from build123d import *

# Parameters (mm, degrees)
SKETCH1_R           = 3.81
BOSS_EXTRUDE1_DEPTH = 17.2974
SKETCH1_6_R         = 3.175
SKETCH1_6_R_2       = 2.8575
CUT_EXTRUDE1_DEPTH  = 2.54
SKETCH1_7_R         = 1.27
CUT_EXTRUDE2_DEPTH  = 1.27


with BuildPart() as part:
    # Sketch1 → Boss-Extrude1 (new body)
    with BuildSketch(Plane.XY):
        Circle(SKETCH1_R)
    extrude(amount=-BOSS_EXTRUDE1_DEPTH)

    # Sketch1<6> → Cut-Extrude1 (cut)
    with BuildSketch(Plane.XY):
        Circle(SKETCH1_6_R)
        Circle(SKETCH1_6_R_2, mode=Mode.SUBTRACT)
    extrude(amount=-CUT_EXTRUDE1_DEPTH, mode=Mode.SUBTRACT)

    # Sketch1<7> → Cut-Extrude2 (cut)
    with BuildSketch(Plane.XY):
        Circle(SKETCH1_7_R)
    extrude(amount=-CUT_EXTRUDE2_DEPTH, mode=Mode.SUBTRACT)


solid = part.part
The model under review builds one solid part; all positions refer to its coordinate system, in mm. A direction names the side the tool comes from. Give positions to 0.01 mm unless a question says otherwise; leave off trailing zeros. Order: outer loops, then holes, each group sorted by start corner. A loop starts at its lowest first (then second) coordinate and runs counter-clockwise, first axis right, second up. Notation, with made-up numbers: M -10,41.5 L -2,41.5 A20 ccw -2,57.5 Z; hole C 20,81.25 d4. An arc over 180 degrees is marked long. Use one line per item in the form item = value. Start each with the question number.
Item 1: For faces 4 (the cylindrical face through (-0.17, 1.26, -0.63)), 5 (the flat face through (0, 0, -17.297)), list the 3-axis set-ups (+Z, -Z, +X, -X, +Y, -Y) from which the entire face can be reached by the end or side of a thin tool; tool diameter is ignored.
Item 2: To check wall thickness, follow line 1 along Y through (x, z) = (0, -0.6) (1 decimal); line 2 along Y through (x, z) = (0, -1.8) (1 decimal); line 3 along Z through (x, y) = (3, -0.5). State the ranges of each line that lie inside material, in increasing order. Write a range as from..to.
Item 3: We need section D-D on x = 2.5. Give the boundary of the cut face in (y, z), plus the area to 3 significant figures.
Item 4: Insertion check: pin 1 Ø2 at (x, z) = (2, -4) entering from -Y; pin 2 Ø4 at (x, z) = (2.5, -6.5) entering from +Y. Each pin has a flat end and moves straight along its axis. Give the tip position at first contact, or say it passes through.
Item 5: The part is to be moulded in two halves that separate along X. For faces 1 (the cylindrical face through (-0.83, -3.72, -8.53)), 2 (the flat face through (-2, 3, 0)), 3 (the cylindrical face through (-0.69, -3.1, -1.25)), say which applies: pulls with the +X half, pulls with the -X half, needs draft (parallel to the pull), parting line crosses it, or undercut.
Item 6: We need section C-C on z = -13. Give the boundary of the cut face in (x, y).
Completed:
q1.face_4 = +Z
q1.face_5 = -Z, +X, -X, +Y, -Y
q2.line_1 = -3.8..-3.2, -2.9..-1.3, 1.3..2.9, 3.2..3.8
q2.line_2 = -3.8..-3.2, -2.9..2.9, 3.2..3.8
q2.line_3 = -17.3..-2.54
q3.outline = M -2.88,-17.3 L 2.88,-17.3 L 2.88,0 L 1.96,0 L 1.96,-2.54 L 1.38,-2.54 L 1.38,0 L -1.38,0 L -1.38,-2.54 L -1.96,-2.54 L -1.96,0 L -2.88,0 Z
q3.area = 96.6 mm²
q4.pin_1 = -3.68
q4.pin_2 = 3.78
q5.face_1 = parting line crosses it
q5.face_2 = needs draft
q5.face_3 = undercut
q6.outline = C 0,0 d7.62
